Work out the finished part from the listing and answer in its coordinate system (mm). A direction names the side the tool comes from. Coordinates: 2 decimals unless noted, no trailing zeros. Loops run counter-clockwise (first coordinate to the right, second up) from the corner with the lowest first, then second, coordinate; pieces in that order, holes last. Notation, with made-up numbers: (48.25, 4) - (77.25, 4) arc R17 ccw to (77.25, 37) - close; hole circle Ø7 at (29.5, 58). An arc over 180 degrees is marked (long way). Write each question's results on one line, items separated by ' | '. Start each with the question number.
Item 1: Section B-B, the plane y = 47 is taken. Write down the section's boundary in (x, z), plus the area to 3 significant figures.
Item 2: For a pull along Y with two mould halves and no side action, classify faces 1 (the face through (5.527, 0.986, 4.665)), 2 (the face through (-9.287, 106.248, 19.036)), 3 (the face through (16.264, 67.752, 11.705)) as +Y half, -Y half, draft (parallel to the pull), parting line (faces both ways), or undercut.
Item 3: Consider probe 1 along X at (y, z) = (54, -2); probe 2 along Z at (x, y) = (10.5, 98.5); probe 3 along Z at (x, y) = (16.1, 64.2). Determine where each line is inside the solid, lowest interval first. Write a range as [from, to].
Item 4: Each of these flat-tipped pins is pushed along its axis until it touches: pin 1 Ø10 at (x, z) = (4, 3) entering from +Y; pin 2 Ø0.6 at (y, z) = (28.5, 18.5) entering from -X; pin 3 Ø2 at (x, z) = (-16, 3.5) entering from +Y. Where does it stop, or does it pass through?
Item 5: A tool of negligible diameter and unlimited length cuts with its end or side. For faces 4 (the face through (-10, 25, -19)), 5 (the face through (16.498, 58.016, 19.337)), 6 (the face through (-16.537, 58.016, 19.298)), 7 (the face through (-16.236, 67.713, 11.666)), 8 (the face through (16, 45, 0)), from which of +Z, -Z, +X, -X, +Y, -Y can it reach the whole face along a straight path? Write none if from no direction.
Item 6: Section C-C, the plane z = -3 is taken. Write down the section's boundary in (x, y).
Item 7: Section A-A, the plane y = 24 is taken. Write down the section's boundary in (x, z), plus the area to 3 significant figures.
Item 8: Section D-D, the plane z = -8 is taken. Count the separate pieces of the cut face and the enclosed holes in it, plus the area to 3 significant figures.
from build123d import *

# Parameters (mm, degrees)
SKETCH2_W           = 34.5
SKETCH2_H           = 40.1
BOSS_EXTRUDE1_DEPTH = 2
SKETCH1_R           = 1
SKETCH1_R_2         = 4.25
CUT_EXTRUDE2_DEPTH  = 3
SKETCH3_W           = 34.5
SKETCH3_H           = 40.1
SKETCH3_W_2         = 30.5
SKETCH3_H_2         = 36.1
BOSS_EXTRUDE3_DEPTH = 110
SKETCH4_W           = 24.336491673
SKETCH4_H           = 45
SKETCH4_H_2         = 40
CUT_EXTRUDE3_DEPTH  = 35.5
SKETCH5_W           = 20
SKETCH5_H           = 40
CUT_EXTRUDE4_DEPTH  = 41.1
FILLET1_R           = 2.5
SKETCH7_R           = 1.350000001
CUT_EXTRUDE5_DEPTH  = 35.5


with BuildPart() as part:
    # Sketch2 → Boss-Extrude1 (new body)
    with BuildSketch(Plane(origin=(0, 0, 0), x_dir=(1, 0, 0), z_dir=(0, 1, 0))):
        Rectangle(SKETCH2_W, SKETCH2_H)
    extrude(amount=BOSS_EXTRUDE1_DEPTH)

    # Sketch1 → Cut-Extrude2 (cut, through all)
    with BuildSketch(Plane(origin=(0, 0, 0), x_dir=(1, 0, 0), z_dir=(0, 1, 0))):
        with Locations((0, 8)):
            Circle(SKETCH1_R)
        with Locations((5.656854249, 5.656854249)):
            Circle(SKETCH1_R)
        with Locations((8, 0)):
            Circle(SKETCH1_R)
        with Locations((5.656854249, -5.656854249)):
            Circle(SKETCH1_R)
        with Locations((0, -8)):
            Circle(SKETCH1_R)
        with Locations((-5.656854249, -5.656854249)):
            Circle(SKETCH1_R)
        with Locations((-8, 0)):
            Circle(SKETCH1_R)
        with Locations((-5.656854249, 5.656854249)):
            Circle(SKETCH1_R)
        Circle(SKETCH1_R_2)
    extrude(amount=CUT_EXTRUDE2_DEPTH, mode=Mode.SUBTRACT)

    # Sketch3 → Boss-Extrude3 (add)
    with BuildSketch(Plane(origin=(0, 2, 0), x_dir=(1, 0, 0), z_dir=(0, 1, 0))):
        Rectangle(SKETCH3_W, SKETCH3_H)
        Rectangle(SKETCH3_W_2, SKETCH3_H_2, mode=Mode.SUBTRACT)
    extrude(amount=BOSS_EXTRUDE3_DEPTH)

    # Sketch4 → Cut-Extrude3 (cut, through all)
    with BuildSketch(Plane.ZY.offset(17.25)):
        with Locations((0.249999999, 89.5)):
            Rectangle(SKETCH4_W, SKETCH4_H)
        with Locations((0.249999999, 25)):
            Rectangle(SKETCH4_W, SKETCH4_H_2)
    extrude(amount=-CUT_EXTRUDE3_DEPTH, mode=Mode.SUBTRACT)

    # Sketch5 → Cut-Extrude4 (cut, through all)
    with BuildSketch(Plane.XY.offset(20.05)):
        with Locations((0, 25)):
            Rectangle(SKETCH5_W, SKETCH5_H)
        with Locations((0, 87)):
            Rectangle(SKETCH5_W, SKETCH5_H)
    extrude(amount=-CUT_EXTRUDE4_DEPTH, mode=Mode.SUBTRACT)

    # Fillet1
    fillet1_edges = [part.edges().sort_by_distance(p)[0] for p in [
        (16.25, 5, -11.918245837),
        (16.25, 45, -11.918245837),
        (16.25, 45, 12.418245836),
        (16.25, 5, 12.418245836),
        (-16.25, 5, -11.918245837),
        (-16.25, 45, -11.918245837),
        (-16.25, 45, 12.418245836),
        (-16.25, 5, 12.418245836),
        (10, 45, -19.05),
        (10, 5, -19.05),
        (-10, 5, -19.05),
        (-10, 45, -19.05),
        (10, 45, 19.05),
        (10, 5, 19.05),
        (-10, 5, 19.05),
        (-10, 45, 19.05),
        (10, 107, -19.05),
        (10, 67, -19.05),
        (-10, 67, -19.05),
        (-10, 107, -19.05),
        (10, 107, 19.05),
        (10, 67, 19.05),
        (-10, 67, 19.05),
        (-10, 107, 19.05),
        (0, 0, 20.05),
        (-17.25, 0, 0),
        (0, 0, -20.05),
        (15.25, 2, 0),
        (0, 2, -18.05),
        (-15.25, 2, 0),
        (0, 2, 18.05),
        (17.25, 0, 0),
        (17.25, 56, 20.05),
        (-17.25, 56, 20.05),
        (-17.25, 56, -20.05),
        (17.25, 56, -20.05),
        (16.25, 67, 12.418245836),
        (16.25, 67, -11.918245837),
        (-16.25, 67, 12.418245836),
        (-16.25, 67, -11.918245837),
    ]]
    fillet(fillet1_edges, radius=FILLET1_R)

    # Sketch7 → Cut-Extrude5 (cut, through all)
    with BuildSketch(Plane.ZY.offset(17.25)):
        with Locations((-14.75, 104.5)):
            Circle(SKETCH7_R)
        with Locations((-14.75, 87.5)):
            Circle(SKETCH7_R)
        with Locations((-14.75, 70.5)):
            Circle(SKETCH7_R)
        with Locations((15.25, 104.5)):
            Circle(SKETCH7_R)
        with Locations((15.25, 87.5)):
            Circle(SKETCH7_R)
        with Locations((15.25, 70.5)):
            Circle(SKETCH7_R)
        with Locations((-8.25, 64.2)):
            Circle(SKETCH7_R)
        with Locations((8.75, 64.2)):
            Circle(SKETCH7_R)
    extrude(amount=-CUT_EXTRUDE5_DEPTH, mode=Mode.SUBTRACT)


solid = part.part
Answer key:
1) outline: (-17.25, -17.55) arc R2.5 ccw to (-14.75, -20.05) - (14.75, -20.05) arc R2.5 ccw to (17.25, -17.55) - (17.25, 17.55) arc R2.5 ccw to (14.75, 20.05) - (-14.75, 20.05) arc R2.5 ccw to (-17.25, 17.55) - close; hole (-15.25, -18.05) - (15.25, -18.05) - (15.25, 18.05) - (-15.25, 18.05) - close | area: 277 mm^2
2) face 1: draft | face 2: undercut | face 3: +Y half
3) probe 1: x = [-17.25, -15.25], [15.25, 17.25] | probe 2: z = [-20.05, -18.05], [18.05, 20.05] | probe 3: z = [-19.65, -9.6], [-6.9, 7.4], [10.1, 19.65]
4) pin 1: stops at y = 2 | pin 2: stops at x = -17.16 | pin 3: stops at y = 67
5) face 4: +Z, -Z | face 5: +Z, +X, +Y, -Y | face 6: +Z, -X, +Y, -Y | face 7: +X, -X, +Y | face 8: +X, -X
6) outline: (-17.25, 2.5) arc R2.5 ccw to (-14.75, 0) - (-3.01, 0) - (-3.01, 2) - (-12.75, 2) arc R2.5 cw to (-15.25, 4.5) - (-15.25, 5) - (-17.25, 5) - close; (-17.25, 45) - (-15.25, 45) - (-15.25, 67) - (-17.25, 67) - close; (3.01, 0) - (14.75, 0) arc R2.5 ccw to (17.25, 2.5) - (17.25, 5) - (15.25, 5) - (15.25, 4.5) arc R2.5 cw to (12.75, 2) - (3.01, 2) - close; (15.25, 45) - (17.25, 45) - (17.25, 67) - (15.25, 67) - close
7) outline: (-17.25, -17.55) arc R2.5 ccw to (-14.75, -20.05) - (-10, -20.05) - (-10, -18.05) - (-15.25, -18.05) - (-15.25, -11.92) - (-17.25, -11.92) - close; (-17.25, 12.42) - (-15.25, 12.42) - (-15.25, 18.05) - (-10, 18.05) - (-10, 20.05) - (-14.75, 20.05) arc R2.5 ccw to (-17.25, 17.55) - close; (10, -20.05) - (14.75, -20.05) arc R2.5 ccw to (17.25, -17.55) - (17.25, -11.92) - (15.25, -11.92) - (15.25, -18.05) - (10, -18.05) - close; (10, 18.05) - (15.25, 18.05) - (15.25, 12.42) - (17.25, 12.42) - (17.25, 17.55) arc R2.5 ccw to (14.75, 20.05) - (10, 20.05) - close | area: 99.7 mm^2
8) separate pieces: 6 | enclosed holes: 0 | area: 154 mm^2
